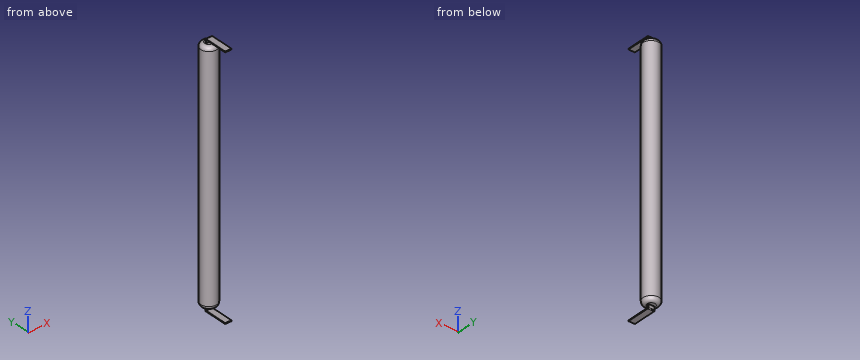
```python
from build123d import *

# Parameters (mm, degrees)
BOSS_EXTRU_1_DEPTH      = 15
BOSS_EXTRU_1_DEPTH_BACK = 15
ESQUISSE1_R             = 1
ESQUISSE2_W             = 0.8
ESQUISSE2_H             = 0.1
BOSS_EXTRU_2_DEPTH      = 1
ESQUISSE3_W             = 0.8
ESQUISSE3_H             = 0.1
BOSS_EXTRU_3_DEPTH      = 1
CONG_1_R                = 0.5
ESQUISSE4_W             = 0.1
ESQUISSE4_H             = 3
BOSS_EXTRU_4_DEPTH      = 0.8
ESQUISSE5_W             = 0.5
ESQUISSE5_H             = 0.1
ENL_V_MAT_EXTRU_1_DEPTH = 0.8
CONG_2_R                = 0.1
ESQUISSE6_W             = 0.1
ESQUISSE6_H             = 3
BOSS_EXTRU_5_DEPTH      = 0.8
ESQUISSE7_W             = 0.5
ESQUISSE7_H             = 0.1
ENL_V_MAT_EXTRU_2_DEPTH = 0.8
CONG_3_R                = 0.1


with BuildPart() as part:
    # Esquisse1 → Boss.-Extru.1 (new, two sides: drawn at the far end of the back side and taken through both)
    with BuildSketch(Plane.XY.offset(-BOSS_EXTRU_1_DEPTH_BACK)):
        Circle(ESQUISSE1_R)
    extrude(amount=BOSS_EXTRU_1_DEPTH + BOSS_EXTRU_1_DEPTH_BACK)

    # Esquisse2 → Boss.-Extru.2 (add)
    with BuildSketch(Plane.XY.offset(15)):
        Rectangle(ESQUISSE2_W, ESQUISSE2_H)
    extrude(amount=BOSS_EXTRU_2_DEPTH)

    # Esquisse3 → Boss.-Extru.3 (add)
    with BuildSketch(Plane(origin=(0, 0, -15), x_dir=(-1, 0, 0), z_dir=(0, 0, -1))):
        Rectangle(ESQUISSE3_W, ESQUISSE3_H)
    extrude(amount=BOSS_EXTRU_3_DEPTH)

    # Congé1
    cong_1_edges = [part.edges().sort_by_distance(p)[0] for p in [
        (-1, 0, 15),
        (-1, 0, -15),
    ]]
    fillet(cong_1_edges, radius=CONG_1_R)

    # Esquisse4 → Boss.-Extru.4 (add)
    with BuildSketch(Plane.ZY.offset(0.4)):
        with Locations((-15.45, -1.45)):
            Rectangle(ESQUISSE4_W, ESQUISSE4_H)
    extrude(amount=-BOSS_EXTRU_4_DEPTH)

    # Esquisse5 → Enlèv. mat.-Extru.1 (cut)
    with BuildSketch(Plane.ZY.offset(0.4)):
        with Locations((-15.75, 0)):
            Rectangle(ESQUISSE5_W, ESQUISSE5_H)
    extrude(amount=-ENL_V_MAT_EXTRU_1_DEPTH, mode=Mode.SUBTRACT)

    # Congé2
    cong_2_edges = [part.edges().sort_by_distance(p)[0] for p in [
        (0, 0.05, -15.5),
    ]]
    fillet(cong_2_edges, radius=CONG_2_R - 0.0001)  # a hair under: the kernel refuses the full size

    # Esquisse6 → Boss.-Extru.5 (add)
    with BuildSketch(Plane.ZY.offset(0.4)):
        with Locations((15.45, -1.45)):
            Rectangle(ESQUISSE6_W, ESQUISSE6_H)
    extrude(amount=-BOSS_EXTRU_5_DEPTH)

    # Esquisse7 → Enlèv. mat.-Extru.2 (cut)
    with BuildSketch(Plane.ZY.offset(0.4)):
        with Locations((15.75, 0)):
            Rectangle(ESQUISSE7_W, ESQUISSE7_H)
    extrude(amount=-ENL_V_MAT_EXTRU_2_DEPTH, mode=Mode.SUBTRACT)

    # Congé3
    cong_3_edges = [part.edges().sort_by_distance(p)[0] for p in [
        (0, 0.05, 15.5),
    ]]
    fillet(cong_3_edges, radius=CONG_3_R)


solid = part.part
```
Work out the finished part from the listing and answer in its coordinate system (mm). Give positions to 0.01 mm unless a question says otherwise; leave off trailing zeros. Order: outer loops, then holes, each group sorted by start corner. A loop starts at its lowest first (then second) coordinate and runs counter-clockwise, first axis right, second up.
1. Section B-B, the plane z = -9 is taken. Determine the outline of the cut face in (x, y).
Result sheet:
outline: circle Ø2 at (0, 0)
2. Straight lines are drawn through the part: L1, parallel to Z at x = -0.3, y = 0.5; L2, parallel to X at y = -0.1, z = 13; L3, parallel to Y at x = 0.8, z = -10. For each, find the intervals that lie inside material, in ascending order.
Result sheet:
L1: z = -14.99 to 14.99
L2: x = -0.99 to 0.99
L3: y = -0.6 to 0.6
3. Section A-A, the plane y = -2.25 is taken. Determine the outline of the cut face in (x, z).
Result sheet:
outline: (-0.4, -15.5) - (0.4, -15.5) - (0.4, -15.4) - (-0.4, -15.4) - close; (-0.4, 15.4) - (0.4, 15.4) - (0.4, 15.5) - (-0.4, 15.5) - close
4. Each of these flat-tipped pins is pushed along its axis until it touches: P1, Ø1, axis at x = 0, z = 12, coming from the -Y side; P2, Ø1.1, axis at x = 0, y = 0, coming from the +Z side. Where does it stop, or does it pass through?
Result sheet:
P1: stops at y = -1
P2: stops at z = 15.5
